Verification items for this drawing (mm, ordinates from the low corner). A direction names the side the tool comes from. Round coordinates to 2 decimals unless told otherwise and drop trailing zeros. Loops run counter-clockwise (first coordinate to the right, second up) from the corner with the lowest first, then second, coordinate; pieces in that order, holes last. Notation, with made-up numbers: (4.25, -21) - (29.25, -21) arc R25 cw to (29.25, 11) - close; hole circle Ø8 at (85, 21). An arc over 180 degrees is marked (long way). Answer in a Markdown table with one row per item. Add a question column.
(1) Cross-section at A-A on x = 50.6. Enter the section's corners in (y, z), then the cut area to 3 significant figures.
(2) Cross-section at D-D on x = 9. Enter the section's corners in (y, z), then the cut area to 3 significant figures.
(3) Access from +Z, -Z, +X, -X, +Y, -Y to the whole of each face (thin tool, end or side, straight path). Record for the marked faces 1, 2, 3 and 4.
(4) Cross-section at C-C on z = 4.2. Enter the section's corners in (x, y), then the cut area to 3 significant figures.
(5) Gauge pin test, flat ends, axial feed: pin 1 (5 mm diameter, centred on x = 50.6, z = 15.8, fed in from -Y); pin 2 (3 mm diameter, centred on y = 36.5, z = 16, fed in from +X); pin 3 (1.6 mm diameter, centred on x = 35.5, y = 38, fed in from +Z). Record the tip position at first contact, or that the pin passes through.
(6) Cross-section at B-B on y = 42. Enter the section's corners in (x, z).
(7) Thickness scan on line 1 along Z through (x, y) = (50.6, 29.95); line 2 along Y through (x, z) = (38.5, 16.25); line 3 along X through (y, z) = (22.5, 4.25). Record the ranges inside material, lowest first.
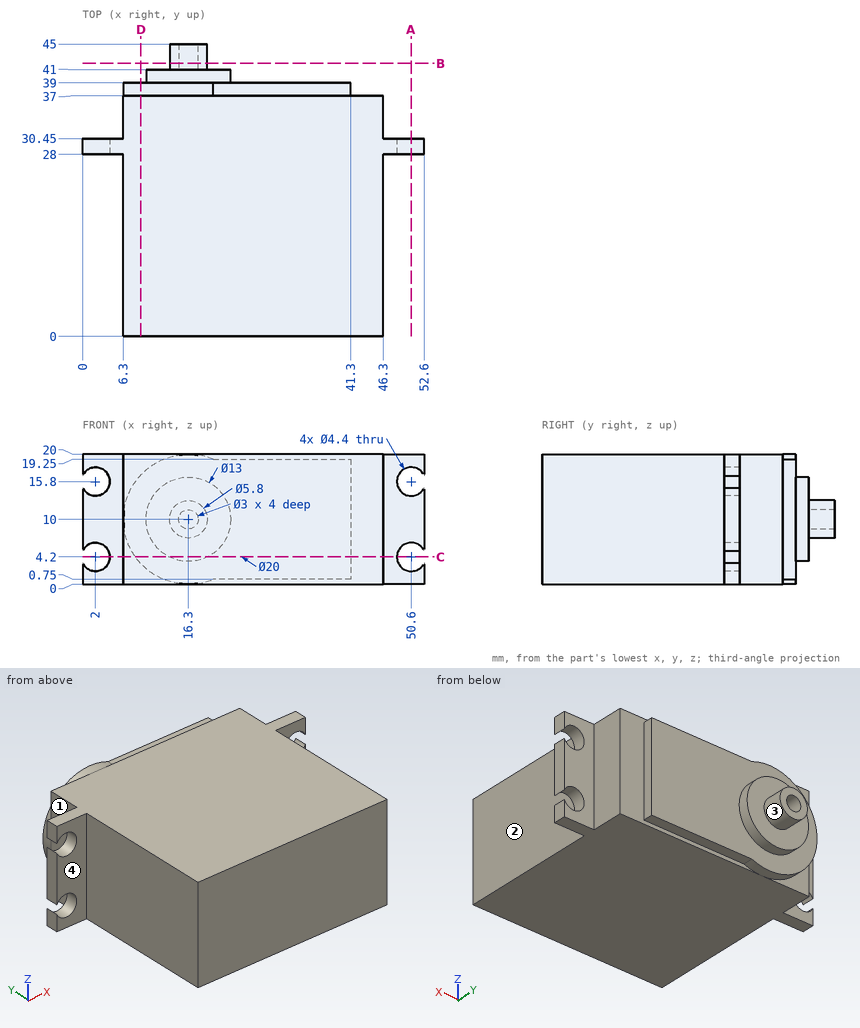
Answers:
| question | item | result |
|---|---|---|
| 1 | outline | (28, 0) - (30.45, 0) - (30.45, 2) - (28, 2) - close; (28, 6.4) - (30.45, 6.4) - (30.45, 13.6) - (28, 13.6) - close; (28, 18) - (30.45, 18) - (30.45, 20) - (28, 20) - close |
| 1 | area | 27.4 mm^2 |
| 2 | outline | (0, 0) - (37, 0) - (37, 3.17) - (39, 3.17) - (39, 16.83) - (37, 16.83) - (37, 20) - (0, 20) - close |
| 2 | area | 767 mm^2 |
| 3 | face 1 | +Z, -Z, -X, +Y |
| 3 | face 2 | +Z, -Z, +X, -Y |
| 3 | face 3 | +Y |
| 3 | face 4 | +Z, -Z, -X, -Y |
| 4 | outline | (4.2, 28) - (6.3, 28) - (6.3, 0) - (46.3, 0) - (46.3, 28) - (48.4, 28) - (48.4, 30.45) - (46.3, 30.45) - (46.3, 37) - (41.3, 37) - (41.3, 39) - (19.23, 39) - (19.23, 41) - (13.37, 41) - (13.37, 39) - (8.15, 39) - (8.15, 37) - (6.3, 37) - (6.3, 30.45) - (4.2, 30.45) - close |
| 4 | area | 1,570 mm^2 |
| 5 | pin 1 | stops at y = 28 |
| 5 | pin 2 | stops at x = 46.3 |
| 5 | pin 3 | stops at z = 19.25 |
| 6 | outline | circle Ø5.8 at (16.3, 10); hole circle Ø3 at (16.3, 10) |
| 7 | line 1 | z = 0 to 2, 6.4 to 13.6, 18 to 20 |
| 7 | line 2 | y = 0 to 39 |
| 7 | line 3 | x = 6.3 to 46.3 |
